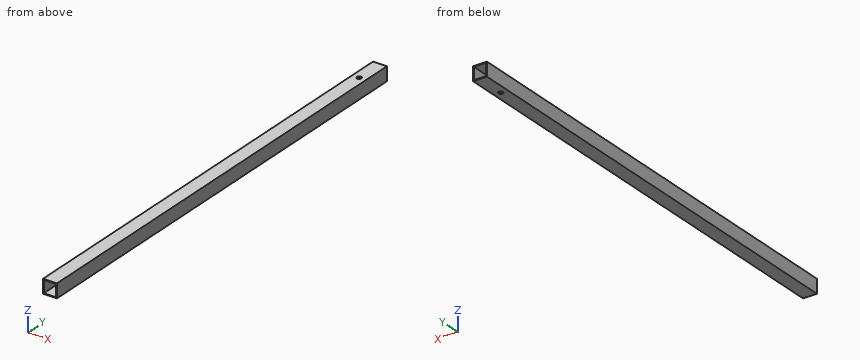
from build123d import *

# Parameters (mm, degrees)
SKETCH1_W           = 18
SKETCH1_H           = 18
SKETCH1_W_2         = 16
SKETCH1_H_2         = 16
BOSS_EXTRUDE1_DEPTH = 600
SKETCH2_R           = 3
CUT_EXTRUDE1_DEPTH  = 993


with BuildPart() as part:
    # Sketch1 → Boss-Extrude1 (new body)
    with BuildSketch(Plane(origin=(0, 0, 0), x_dir=(1, 0, 0), z_dir=(0, 1, 0))):
        Rectangle(SKETCH1_W, SKETCH1_H)
        Rectangle(SKETCH1_W_2, SKETCH1_H_2, mode=Mode.SUBTRACT)
    extrude(amount=BOSS_EXTRUDE1_DEPTH)

    # Sketch2 → Cut-Extrude1 (cut)
    with BuildSketch(Plane.XY.offset(9)):
        with Locations((0, 562)):
            Circle(SKETCH2_R)
    extrude(amount=-CUT_EXTRUDE1_DEPTH, mode=Mode.SUBTRACT)


solid = part.part
Can you work these out from the model? Positions are in its coordinate system, mm. Give positions to 0.01 mm unless a question says otherwise; leave off trailing zeros. Loops run counter-clockwise (first coordinate to the right, second up) from the corner with the lowest first, then second, coordinate; pieces in that order, holes last. Notation, with made-up numbers: (-18.5, 63.5) -> (17.5, 63.5) arc R24 ccw to (17.5, 74.5) -> close; hole circle Ø9 at (-15.5, -38.5). An arc over 180 degrees is marked (long way). Write item = value, one per line.
1) I need wall thicknesses on L1, parallel to X at y = 366.5, z = 3; L2, parallel to Y at x = 0, z = -8.15. Which ranges of each line are inside material? Lowest first, please. Write a range as from..to.
Check result:
L1 = -9..-8, 8..9
L2 = 0..559, 565..600
2) Suppose I cut it at B-B on x = 0. Write out the boundary of the cut face in (y, z).
Check result:
outline = (0, -9) -> (559, -9) -> (559, -8) -> (0, -8) -> close; (0, 8) -> (559, 8) -> (559, 9) -> (0, 9) -> close; (565, -9) -> (600, -9) -> (600, -8) -> (565, -8) -> close; (565, 8) -> (600, 8) -> (600, 9) -> (565, 9) -> close
3) Suppose I cut it at A-A on z = -0.5. Write out the boundary of the cut face in (x, y), then the cut area to 3 significant figures.
Check result:
outline = (-9, 0) -> (-8, 0) -> (-8, 600) -> (-9, 600) -> close; (8, 0) -> (9, 0) -> (9, 600) -> (8, 600) -> close
area = 1,200 mm2
4) Suppose I cut it at C-C on y = 323. Write out the boundary of the cut face in (x, z).
Check result:
outline = (-9, -9) -> (9, -9) -> (9, 9) -> (-9, 9) -> close; hole (-8, -8) -> (8, -8) -> (8, 8) -> (-8, 8) -> close
